Model file for the job. Use its own axes, mm. A direction names the side the tool comes from. Coordinates: 2 decimals unless noted, no trailing zeros. Order: outer loops, then holes, each group sorted by start corner. A loop starts at its lowest first (then second) coordinate and runs counter-clockwise, first axis right, second up. Notation, with made-up numbers: M 0.5,76.5 L 21.5,76.5 A18 cw 21.5,94.5 Z; hole C 32,17 d11. An arc over 180 degrees is marked long. Return JSON: item names as keys, results as strings.
```python
from build123d import *

# Parameters (mm, degrees)
SKETCH1_W                  = 6.54
SKETCH1_H                  = 6.095
EXTRUDE1_DEPTH             = 1.1425
EXTRUDE1_TAPER             = 7.5
EXTRUDE1_OTHER_WAY_DEPTH   = 1.1425
EXTRUDE1_OTHER_WAY_TAPER   = 7.5
EXTRUDE2_REACH             = 6.614
EXTRUDE2_DIRECTION_2_REACH = 6.614
CUT_EXTRUDE5_REACH         = 7.74
EXTRUDE5_DEPTH             = 0.3825
SKETCH29_W                 = 1.02
SKETCH29_H                 = 0.535
EXTRUDE6_DEPTH             = 0.3825


with BuildPart() as part:
    # Sketch1 → Extrude1 (new body)
    with BuildSketch(Plane(origin=(0, 0, 0), x_dir=(1, 0, 0), z_dir=(0, 1, 0))):
        Rectangle(SKETCH1_W, SKETCH1_H)
    extrude(amount=EXTRUDE1_DEPTH, taper=EXTRUDE1_TAPER)

    # Sketch1 → Extrude1 other way (add)
    with BuildSketch(Plane(origin=(0, 0, 0), x_dir=(1, 0, 0), z_dir=(0, 1, 0))):
        Rectangle(SKETCH1_W, SKETCH1_H)
    extrude(amount=-EXTRUDE1_OTHER_WAY_DEPTH, taper=EXTRUDE1_OTHER_WAY_TAPER)

    # Extrude2: up to this plane
    extrude2_end = Plane(origin=(3.27, 0, -3.0475), z_dir=(0.9914448613738104, -0.13052619222005188, 0))
    # Sketch2 → Extrude2 (add, up to the surface)
    with BuildSketch(Plane(origin=(0, 0, 0), x_dir=(0, 0, -1), z_dir=(1, 0, 0)), mode=Mode.PRIVATE) as extrude2_sk1:
        Polygon((3.0475, 0), (2.897087022, -1.1425), (4.1275, -1.1425), (4.1275, -0.4675), (3.109047543, -0.4675), align=None)
    extrude2_tool1 = split(extrude(extrude2_sk1.sketch, amount=EXTRUDE2_REACH, mode=Mode.PRIVATE), bisect_by=extrude2_end, keep=Keep.BOTH, mode=Mode.PRIVATE)
    add(extrude2_tool1.solids().sort_by_distance((0, -0.791952, -3.517345))[0])

    # Extrude2 direction 2: up to this plane
    extrude2_direction_2_end = Plane(origin=(-3.27, 0, -3.0475), z_dir=(-0.9914448613738104, -0.13052619222005188, 0))
    # Sketch2 → Extrude2 direction 2 (add, up to the surface)
    with BuildSketch(Plane(origin=(0, 0, 0), x_dir=(0, 0, -1), z_dir=(1, 0, 0)), mode=Mode.PRIVATE) as extrude2_direction_2_sk1:
        Polygon((3.0475, 0), (2.897087022, -1.1425), (4.1275, -1.1425), (4.1275, -0.4675), (3.109047543, -0.4675), align=None)
    extrude2_direction_2_tool1 = split(extrude(extrude2_direction_2_sk1.sketch, amount=-EXTRUDE2_DIRECTION_2_REACH, mode=Mode.PRIVATE), bisect_by=extrude2_direction_2_end, keep=Keep.BOTH, mode=Mode.PRIVATE)
    add(extrude2_direction_2_tool1.solids().sort_by_distance((0, -0.791952, -3.517345))[0])

    # Sketch27 → Cut-Extrude5 (cut, up to next)
    with BuildSketch(Plane(origin=(0, 1.1425, 0), x_dir=(1, 0, 0), z_dir=(0, 1, 0)), mode=Mode.PRIVATE) as cut_extrude5_sk1:
        with BuildLine():
            Line((2.6025, 3.109047543), (2.6025, 3.896559892))
            Line((2.6025, 3.896559892), (2.2025, 4.1275))
            Line((2.2025, 4.1275), (3.27, 4.1275))
            Line((3.27, 4.1275), (3.27, 2.441547543))
            ThreePointArc((3.27, 2.441547543), (2.798006224, 2.637053766), (2.6025, 3.109047543))
        make_face()
    cut_extrude5_tool1 = extrude(cut_extrude5_sk1.sketch, amount=-CUT_EXTRUDE5_REACH, mode=Mode.PRIVATE) & part.part
    # Sketch27 → Cut-Extrude5 (cut, up to next)
    with BuildSketch(Plane(origin=(0, 1.1425, 0), x_dir=(1, 0, 0), z_dir=(0, 1, 0)), mode=Mode.PRIVATE) as cut_extrude5_sk2:
        with BuildLine():
            Line((-2.6025, 3.896559892), (-2.2025, 4.1275))
            Line((-2.2025, 4.1275), (-3.27, 4.1275))
            Line((-3.27, 4.1275), (-3.27, 2.441547543))
            ThreePointArc((-3.27, 2.441547543), (-2.798006224, 2.637053766), (-2.6025, 3.109047543))
            Line((-2.6025, 3.109047543), (-2.6025, 3.896559892))
        make_face()
    cut_extrude5_tool2 = extrude(cut_extrude5_sk2.sketch, amount=-CUT_EXTRUDE5_REACH, mode=Mode.PRIVATE) & part.part
    add(cut_extrude5_tool1.solids().sort_by_distance((2.932609, 1.1425, -3.37907))[0], mode=Mode.SUBTRACT)
    add(cut_extrude5_tool2.solids().sort_by_distance((-2.932609, 1.1425, -3.37907))[0], mode=Mode.SUBTRACT)

    # Sketch28 → Extrude5 (add, symmetric)
    with BuildSketch(Plane(origin=(2.29, 0, 0), x_dir=(0, 0, -1), z_dir=(1, 0, 0))):
        with BuildLine():
            Line((-2.977065914, 0.535), (-3.477818827, 0.535))
            ThreePointArc((-3.477818827, 0.535), (-3.993129319, 0.401312635), (-4.378457731, 0.033971882))
            Line((-4.378457731, 0.033971882), (-4.663971185, -0.426059351))
            ThreePointArc((-4.663971185, -0.426059351), (-4.836678027, -0.598050142), (-5.068098093, -0.6745566))
            Line((-5.068098093, -0.6745566), (-5.810814161, -0.739535837))
            Line((-5.810814161, -0.739535837), (-5.764185839, -1.2725))
            Line((-5.764185839, -1.2725), (-5.018976864, -1.207302663))
            ThreePointArc((-5.018976864, -1.207302663), (-4.556136732, -1.054289745), (-4.210723048, -0.710308165))
            Line((-4.210723048, -0.710308165), (-3.925356764, -0.250514059))
            ThreePointArc((-3.925356764, -0.250514059), (-3.732692558, -0.066843683), (-3.475037312, 0))
            Line((-3.475037312, 0), (-2.977065914, 0))
            Line((-2.977065914, 0), (-2.977065914, 0.535))
        make_face()
    extrude5 = extrude(amount=EXTRUDE5_DEPTH, both=True)

    # Sketch29 → Extrude6 (add, symmetric)
    with BuildSketch(Plane(origin=(0, 0, 0), x_dir=(0, 0, -1), z_dir=(1, 0, 0))):
        with Locations((-3.487065914, 0.2675)):
            Rectangle(SKETCH29_W, SKETCH29_H)
    extrude(amount=EXTRUDE6_DEPTH, both=True)

    # Mirror1: Extrude5 across plane
    add(extrude5.mirror(Plane(origin=(0, 0, 0), x_dir=(0, 0, 1), z_dir=(1, 0, 0))))


solid = part.part
```
Item 1: Saw through at B-B (y = -1). Count the separate pieces of the cut face and the enclosed holes in it, and give its area (3 significant figures).
Check result:
{"separate pieces": "3", "enclosed holes": "0", "area": "44.5 mm2"}
Item 2: 3-axis set-ups, long thin cutter, end or side, ignore diameter. For faces 1 (the flat face through (0, -1.142, -1)), 2 (the flat face through (0, 1.142, 0)): which of +Z, -Z, +X, -X, +Y, -Y reach the whole face in a straight line?
Check result:
{"face 1": "-Z, +X, -X, -Y", "face 2": "+Z, -Z, +X, -X, +Y"}
Item 3: Wall check: line 1 (X direction, y = -0.85, z = 4.5); line 2 (Y direction, x = -0.75, z = 2); line 3 (Z direction, x = 2, y = -0.6). Give the ranges that are in metal, low to high.
Check result:
{"line 1": "x = -2.67 to -1.91, 1.91 to 2.67", "line 2": "y = -1.14 to 1.14", "line 3": "z = -4.13 to 2.97, 4.14 to 4.84"}
Item 4: Pull direction X, two halves, no side cores. Call faces 3 (the flat face through (1.908, 0, 4)), 4 (the flat face through (0, -0.468, -3.6)), 5 (the flat face through (-1.908, 0, 4)), 6 (the flat face through (-3.196, -0.563, 0.333)): +X half, -X half, draft (parallel to the pull), parting line (faces both ways), or undercut.
Check result:
{"face 3": "undercut", "face 4": "draft", "face 5": "undercut", "face 6": "-X half"}
Item 5: Drop flat-ended pins along their axis: pin 1 Ø0.5 at (y, z) = (-0.5, -3.5) entering from +X; pin 2 Ø0.6 at (x, z) = (0, 3.5) entering from +Y (3 decimals); pin 3 Ø0.9 at (y, z) = (0, 4) entering from -X. Give the stop position or say it passes through.
Check result:
{"pin 1": "stops at x = 2.6", "pin 2": "stops at y = 0.535", "pin 3": "stops at x = -2.67"}
Item 6: Saw through at A-A (z = -3.5). Write the cut outline in (x, y).
Check result:
{"outline": "M -2.6,-1.14 L 2.6,-1.14 L 2.6,-0.47 L -2.6,-0.47 Z"}
